Check sheet for the drawn part. Datum: minimum x, y, z corner. Units: mm. Round coordinates to 2 decimals unless told otherwise and drop trailing zeros. Write each loop counter-clockwise with the first axis right and the second up, starting at its lowest first coordinate (ties: lowest second). Pieces come first, ordered by that corner, then holes.
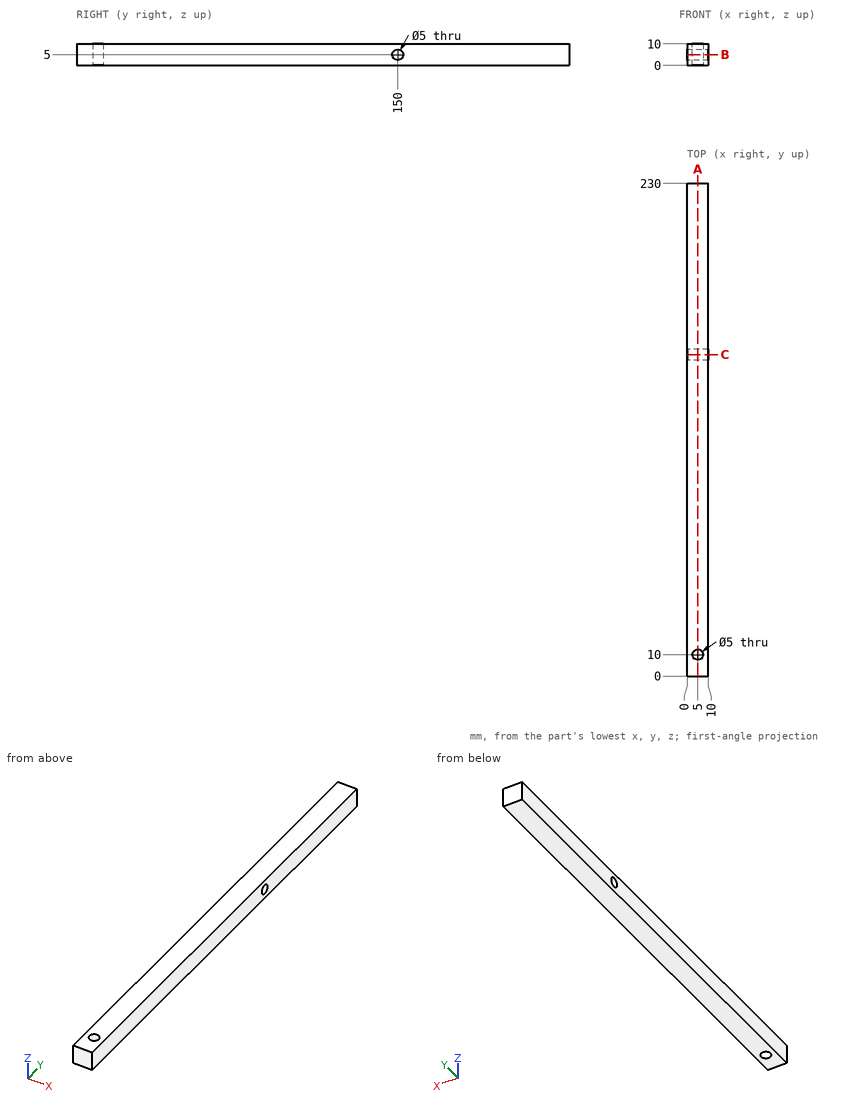
1. Sectioned sample at C-C, the plane y = 150. Enter the section's corners in (x, z), plus the area to 3 significant figures.
2. Go/stop test with flat-tipped pins: pin 1 (3 mm diameter, centred on y = 81, z = 4.5, fed in from -X); pin 2 (4.5 mm diameter, centred on x = 5, y = 10, fed in from +Z). Record where each tip stops, or that it passes through.
3. Scan lines: line 1 along Y through (x, z) = (5, 5.5); line 2 along Y through (x, z) = (6.5, 5.75); line 3 along Z through (x, y) = (3.5, 150). Record each from-to range of solid material in increasing order.
4. Sectioned sample at A-A, the plane x = 5. Enter the section's corners in (y, z), plus the area to 3 significant figures.
5. Sectioned sample at B-B, the plane z = 5. Enter the section's corners in (x, y).
Computed values:
1. outline: (0, 0) - (10, 0) - (10, 2.5) - (0, 2.5) - close; (0, 7.5) - (10, 7.5) - (10, 10) - (0, 10) - close
1. area: 50.0 mm2
2. pin 1: stops at x = 0
2. pin 2: passes through
3. line 1: y = 0 to 7.5, 12.5 to 147.55, 152.45 to 230
3. line 2: y = 0 to 8, 12 to 147.62, 152.38 to 230
3. line 3: z = 0 to 2.5, 7.5 to 10
4. outline: (0, 0) - (7.5, 0) - (7.5, 10) - (0, 10) - close; (12.5, 0) - (230, 0) - (230, 10) - (12.5, 10) - close; hole circle Ø5 at (150, 5)
4. area: 2,230 mm2
5. outline: (0, 0) - (10, 0) - (10, 147.5) - (0, 147.5) - close; (0, 152.5) - (10, 152.5) - (10, 230) - (0, 230) - close; hole circle Ø5 at (5, 10)
